```python
from build123d import *

# Parameters (mm, degrees)
F0_R     = 3.5
F1_DEPTH = 5
F3_START = 2
F2_R     = 2.625
F2_R_2   = 0.75
F3_DEPTH = 3


with BuildPart() as f1:
    # F0 (on Top) → F1 (new body)
    with BuildSketch(Plane.XY):
        Circle(F0_R)
    extrude(amount=F1_DEPTH)

    # F2 (on Top) → F3 (cut)
    with BuildSketch(Plane.XY.offset(F3_START)):
        Circle(F2_R)
        Circle(F2_R_2, mode=Mode.SUBTRACT)
    extrude(amount=F3_DEPTH, mode=Mode.SUBTRACT)


solid = f1.part
```
For this review, take the finished solid that the model builds, in its own axes (mm). A direction names the side the tool comes from. Coordinates: 2 decimals unless noted, no trailing zeros. Write each loop counter-clockwise with the first axis right and the second up, starting at its lowest first coordinate (ties: lowest second). Pieces come first, ordered by that corner, then holes. Notation, with made-up numbers: (12, 11.5) -> (20, 11.5) arc R17 cw to (20, 42.5) -> close; hole circle Ø4 at (72.5, 21). An arc over 180 degrees is marked (long way). Put each result on its own line as item: value.
Q1. Take a section at B-B, the plane y = 0. State the section outline as (x, z) points (3 decimals).
From the geometry:
outline: (-3.5, 0) -> (3.5, 0) -> (3.5, 5) -> (2.625, 5) -> (2.625, 2) -> (0.75, 2) -> (0.75, 5) -> (-0.75, 5) -> (-0.75, 2) -> (-2.625, 2) -> (-2.625, 5) -> (-3.5, 5) -> close
Q2. Take a section at A-A, the plane z = 4.6. State the section outline as (x, y) points (3 decimals).
From the geometry:
outline: circle Ø7 at (0, 0); circle Ø1.5 at (0, 0); hole circle Ø5.25 at (0, 0)
Q3. The part is to be moulded in two halves that separate along X. For faces 1 (the flat face through (1, -1, 2)), 2 (the cylindrical face through (3.233, -1.341, 2.465)), 3 (the flat face through (0, 0, 5)), say which applies: +X half, -X half, draft (parallel to the pull), parting line (faces both ways), or undercut.
From the geometry:
face 1: undercut
face 2: parting line
face 3: draft
Q4. Wall thickness on L1, parallel to Y at x = 0, z = 3.9 (3 decimals); L2, parallel to Y at x = -1.5, z = 2.05; L3, parallel to Z at x = 0.75, y = 0.75: over which ranges is each line inside the solid? List them lowest first.
From the geometry:
L1: y = -3.5 to -2.625, -0.75 to 0.75, 2.625 to 3.5
L2: y = -3.16 to -2.15, 2.15 to 3.16
L3: z = 0 to 2
Q5. Take a section at D-D, the plane x = -2.5. State the section outline as (y, z) points, then the cut area to 3 significant figures.
From the geometry:
outline: (-2.45, 0) -> (2.45, 0) -> (2.45, 5) -> (0.8, 5) -> (0.8, 2) -> (-0.8, 2) -> (-0.8, 5) -> (-2.45, 5) -> close
area: 19.7 mm2
Q6. Tool access review of faces 4 (the flat face through (1, 3, 5)), 5 (the cylindrical face through (-0.75, 0.03, 3.48)): name each direction out of +Z, -Z, +X, -X, +Y, -Y from which nothing blocks a thin tool from reaching the whole face with its end or side.
From the geometry:
face 4: +Z, +X, -X, +Y, -Y
face 5: +Z
Q7. Clearance check with flat-ended pins moving along their axes: pin 1 Ø4 at (x, y) = (2, 2.5) entering from -Z; pin 2 Ø1.5 at (y, z) = (-1, 4) entering from -X; pin 3 Ø1.5 at (x, z) = (1.5, 4) entering from -Y; pin 4 Ø3 at (x, z) = (2.5, 2) entering from +Y. State where each tip first meets the part, or that it passes through.
From the geometry:
pin 1: stops at z = 0
pin 2: stops at x = -3.49
pin 3: stops at y = -3.42
pin 4: stops at y = 3.35
